```python
from build123d import *

# Parameters (mm, degrees)
SKETCH_1_W          = 25
SKETCH_1_H          = 20
EXTRUDE_1_DEPTH     = 100
SKETCH_2_R          = 5.2
CUT_EXTRUDE_1_DEPTH = 8
SKETCH_3_W          = 2
SKETCH_3_H          = 20
EXTRUDE_2_DEPTH     = 10
EXTRUDE_3_DEPTH     = 20
SKETCH_6_R          = 1.6
CUT_EXTRUDE_2_DEPTH = 3
SKETCH_7_W          = 2
SKETCH_7_H          = 20
EXTRUDE_4_DEPTH     = 10
EXTRUDE_5_DEPTH     = 20
SKETCH_9_R          = 1.6
CUT_EXTRUDE_3_DEPTH = 3


with BuildPart() as part:
    # ｽｹｯﾁ1 → ﾎﾞｽ - 押し出し1 (new body)
    with BuildSketch(Plane.XY):
        with Locations((-0.22894462, -4.808467742)):
            Rectangle(SKETCH_1_W, SKETCH_1_H)
    extrude(amount=EXTRUDE_1_DEPTH)

    # ｽｹｯﾁ2 → ｶｯﾄ - 押し出し1 (cut)
    with BuildSketch(Plane(origin=(0, 5.191532258, 0), x_dir=(1, 0, 0), z_dir=(0, 1, 0))):
        with Locations((-0.22894462, -90)):
            Circle(SKETCH_2_R)
    extrude(amount=-CUT_EXTRUDE_1_DEPTH, mode=Mode.SUBTRACT)

    # ｽｹｯﾁ3 → ﾎﾞｽ - 押し出し2 (add)
    with BuildSketch(Plane(origin=(12.27105538, 0, 0), x_dir=(0, 0, -1), z_dir=(1, 0, 0))):
        with Locations((-1, -4.808467742)):
            Rectangle(SKETCH_3_W, SKETCH_3_H)
    extrude(amount=EXTRUDE_2_DEPTH)

    # ｽｹｯﾁ5 → ﾎﾞｽ - 押し出し3 (add, through all)
    with BuildSketch(Plane(origin=(0, 5.191532258, 0), x_dir=(1, 0, 0), z_dir=(0, 1, 0))):
        Polygon((12.27105538, -5), (15.27105538, -2), (12.27105538, -2), align=None)
    extrude(amount=-EXTRUDE_3_DEPTH)

    # ｽｹｯﾁ6 → ｶｯﾄ - 押し出し2 (cut, through all)
    with BuildSketch(Plane.XY.offset(2)):
        with Locations((18.77105538, 1.691532258)):
            Circle(SKETCH_6_R)
        with Locations((18.77105538, -11.308467742)):
            Circle(SKETCH_6_R)
    extrude(amount=-CUT_EXTRUDE_2_DEPTH, mode=Mode.SUBTRACT)

    # ｽｹｯﾁ7 → ﾎﾞｽ - 押し出し4 (add)
    with BuildSketch(Plane.ZY.offset(12.72894462)):
        with Locations((1, -4.808467742)):
            Rectangle(SKETCH_7_W, SKETCH_7_H)
    extrude(amount=EXTRUDE_4_DEPTH)

    # ｽｹｯﾁ8 → ﾎﾞｽ - 押し出し5 (add, through all)
    with BuildSketch(Plane.XZ.offset(14.808467742)):
        Polygon((-12.72894462, 5), (-15.72894462, 2), (-12.72894462, 2), align=None)
    extrude(amount=-EXTRUDE_5_DEPTH)

    # ｽｹｯﾁ9 → ｶｯﾄ - 押し出し3 (cut, through all)
    with BuildSketch(Plane.XY.offset(2)):
        with Locations((-19.22894462, -11.308467742)):
            Circle(SKETCH_9_R)
        with Locations((-19.22894462, 1.691532258)):
            Circle(SKETCH_9_R)
    extrude(amount=-CUT_EXTRUDE_3_DEPTH, mode=Mode.SUBTRACT)


solid = part.part
```
Geometry: final body of the model. Coordinates: model frame, mm. A direction names the side the tool comes from. Coordinates: 2 decimals unless noted, no trailing zeros. Order: outer loops, then holes, each group sorted by start corner. A loop starts at its lowest first (then second) coordinate and runs counter-clockwise, first axis right, second up. Notation, with made-up numbers: (8, -4) -> (50, -4) arc R31 ccw to (50, 22) -> close; hole circle Ø6 at (0.25, 80.25). An arc over 180 degrees is marked (long way). Write each question's results on one line, items separated by ' | '. Start each with the question number.
1) First-contact query: pin 1 (8 mm diameter, centred on y = -3, z = 48.5, fed in from +X); pin 2 (1.9 mm diameter, centred on x = 18.77, y = 1.69, fed in from +Z); pin 3 (2 mm diameter, centred on x = 19, y = -5.5, fed in from +Z); pin 4 (12 mm diameter, centred on y = 0, z = 78, fed in from -X). Flat tips, straight axial feed; report the tip coordinate or a pass-through.
2) Material intervals for line 1 along X through (y, z) = (-1, 90); line 2 along X through (y, z) = (3.75, 16); line 3 along Z through (x, y) = (16, -8), sorted ascending.
3) Cut plane C-C, the plane x = -2. Output: boundary loops of the cut face in (y, z), and give its area (3 significant figures).
4) Cut plane D-D, the plane z = 53. Output: boundary loops of the cut face in (x, y), and give its area (3 significant figures).
5) Cut plane B-B, the plane y = -3.75. Output: boundary loops of the cut face in (x, z), and give its area (3 significant figures).
6) Set-up query: faces 4 (the flat face through (19, -5, 2)), 5 (the flat face through (0, -2.808, 90)), 6 (the flat face through (-19, -5, 2)). Return all of +Z, -Z, +X, -X, +Y, -Y with unobstructed straight access to the full face (end or side cutting, diameter ignored); none if empty.
7) Cut plane A-A, the plane z = 90. Output: boundary loops of the cut face in (x, y), and give its area (3 significant figures).
8) Mould query, pull axis Z, two halves, no side actions, for faces 1 (the flat face through (13.75, -4.67, 3.52)), 2 (the flat face through (-1, -14.808, 51)), 3 (the cylindrical face through (-1.356, 1.248, 95.076)). Classes: released by +Z, released by -Z, zero draft, split by the parting line, or undercut.
Checks:
1) pin 1: x = 12.27 | pin 2: through | pin 3: z = 2 | pin 4: x = -12.73
2) line 1: -12.73 to -5.43, 4.97 to 12.27 | line 2: -12.73 to 12.27 | line 3: 0 to 2
3) outline: (-14.81, 0) -> (5.19, 0) -> (5.19, 85.11) -> (-2.81, 85.11) -> (-2.81, 94.89) -> (5.19, 94.89) -> (5.19, 100) -> (-14.81, 100) -> close | area: 1,920 mm^2
4) outline: (-12.73, -14.81) -> (12.27, -14.81) -> (12.27, 5.19) -> (-12.73, 5.19) -> close | area: 500 mm^2
5) outline: (-22.73, 0) -> (22.27, 0) -> (22.27, 2) -> (15.27, 2) -> (12.27, 5) -> (12.27, 100) -> (-12.73, 100) -> (-12.73, 5) -> (-15.73, 2) -> (-22.73, 2) -> close | area: 2,550 mm^2
6) face 4: +Z, +X, +Y, -Y | face 5: +Y | face 6: +Z, -X, +Y, -Y
7) outline: (-12.73, -14.81) -> (12.27, -14.81) -> (12.27, 5.19) -> (4.97, 5.19) -> (4.97, -2.81) -> (-5.43, -2.81) -> (-5.43, 5.19) -> (-12.73, 5.19) -> close | area: 417 mm^2
8) face 1: released by +Z | face 2: zero draft | face 3: undercut
